from build123d import *

# Parameters (mm, degrees)
F1_DEPTH = 63.5
F0_W     = 25.4
F0_H     = 19.05
F2_DEPTH = 25.4
F3_DEPTH = 7.9375
F5_R     = 5.08


with BuildPart() as f1:
    # F0 (on Front) → F1 (new body, symmetric)
    with BuildSketch(Plane.XZ):
        Polygon((41.275, -9.525), (41.275, 9.525), (22.225, 9.525), (-41.275, 9.525), (-41.275, -9.525), align=None)
    extrude(amount=F1_DEPTH, both=True)

    # F0 (on Front) → F2 (join, symmetric)
    with BuildSketch(Plane.XZ):
        with BuildLine():
            Line((22.225, 9.525), (41.275, 9.525))
            Line((41.275, 9.525), (41.275, 27.0666779783))
            ThreePointArc((41.275, 27.0666779783), (45.3781164095, 37.7174235733), (55.566449667, 42.8625))
            Line((55.566449667, 42.8625), (60.325, 42.8625))
            Line((60.325, 42.8625), (60.325, 61.9125))
            Line((60.325, 61.9125), (54.799614366, 61.9125))
            ThreePointArc((54.799614366, 61.9125), (31.6368382666, 50.9169233306), (22.225, 27.0666779783))
            Line((22.225, 27.0666779783), (22.225, 9.525))
        make_face()
        with Locations((73.025, 52.3875)):
            Rectangle(F0_W, F0_H)
    extrude(amount=F2_DEPTH, both=True)

    # F0 (on Front) → F3 (join, symmetric)
    with BuildSketch(Plane.XZ):
        with BuildLine():
            Line((-41.275, 9.525), (22.225, 9.525))
            Line((22.225, 9.525), (22.225, 27.0666779783))
            ThreePointArc((22.225, 27.0666779783), (31.6368382666, 50.9169233306), (54.799614366, 61.9125))
            add(Edge.make_bspline(
                [(-41.275, 9.525), (-33.6213931441, 35.8969122171), (10.3490389884, 59.2281594872), (54.799614366, 61.9125)],
                knots=[0, 0, 0, 0, 109.4293456154, 109.4293456154, 109.4293456154, 109.4293456154], degree=3))
        make_face()
    extrude(amount=F3_DEPTH, both=True)

    # F0 (on Front) → F4 (revolve)
    with BuildSketch(Plane.XZ):
        Polygon((85.725, 61.9125), (85.725, 42.8625), (85.725, 37.1208467424), (111.125, 37.1208467424), (111.125, 65.6958467424), (85.725, 65.6958467424), align=None)
    revolve(axis=Axis((85.725, 0, 51.4083467424), (0, 0, 1)))

    # F5
    f5_edges = [f1.edges().sort_by_distance(p)[0] for p in [
        (41.275, -63.5, 0),
        (41.275, 63.5, 0),
        (-41.275, -63.5, 0),
        (-41.275, 63.5, 0),
        (41.275, 0, 27.066678),
    ]]
    fillet(f5_edges, radius=F5_R)


solid = f1.part
Could you check a few things on this model? Use its own coordinates, in mm. A direction names the side the tool comes from. Coordinates: 2 decimals unless noted, no trailing zeros. Order: outer loops, then holes, each group sorted by start corner. A loop starts at its lowest first (then second) coordinate and runs counter-clockwise, first axis right, second up. Notation, with made-up numbers: (36.5, 22) - (62.5, 22) arc R24 ccw to (62.5, 32) - close; hole circle Ø11 at (-32.5, -2). An arc over 180 degrees is marked (long way). Answer in a Markdown table with one row per item. Add a question column.
(1) On a 3-axis mill with a long thin cutter (end or side, diameter ignored), from which of +Z, -Z, +X, -X, +Y, -Y can I reach the whole of each face in a straight line? I mean faces 4 (the face through (-5, -7.938, 30)), 5 (the face through (60, 0, 61.912)), 6 (the face through (86, 0, 37.121)), 7 (the face through (22.225, 17, 18)), 8 (the face through (45.269, -0.356, 37.596)). Say none if no direction works.
(2) If we section it at C-C, the plane y = -42.5: Please give me the cut outline in (x, z) (3 decimals), then the cut area to 3 significant figures.
(3) If we section it at A-A, the plane z = -3: Please give me the cut outline in (x, y) (3 decimals).
(4) I need wall thicknesses on L1, parallel to Z at x = 67, y = -3; L2, parallel to Y at x = 11, z = 49; L3, parallel to Y at x = 34, z = 32. Which ranges of each line are inside material? Lowest first, please.
(5) Will these pins go through, and if not, where does the flat tip stop? pin 1 (15.5 mm diameter, centred on x = 22.5, z = 41, fed in from +Y); pin 2 (5 mm diameter, centred on x = -22.5, y = 34.5, fed in from +Z) (3 decimals); pin 3 (19 mm diameter, centred on y = -18, z = 20, fed in from -X) (3 decimals).
(6) If we mould it in two halves opening along X, with no side actions, what happens to faces 1 (the face through (39.8, -62, 0.1)), 2 (the face through (59, 0, 42.862)), 3 (the face through (46, 25.4, 42))? For each: released by +X, released by -X, zero draft, split by the parting line, or undercut.
Results are:
| question | item | result |
|---|---|---|
| 1 | face 4 | +Z, -X, -Y |
| 1 | face 5 | +Z, -X |
| 1 | face 6 | -Z, +X, +Y, -Y |
| 1 | face 7 | +Z, -X, +Y |
| 1 | face 8 | -Z, +Y, -Y |
| 2 | outline | (-41.275, -9.525) - (41.275, -9.525) - (41.275, 9.525) - (-41.275, 9.525) - close |
| 2 | area | 1,570 mm2 |
| 3 | outline | (-41.275, -58.42) arc R5.08 ccw to (-36.195, -63.5) - (36.195, -63.5) arc R5.08 ccw to (41.275, -58.42) - (41.275, 58.42) arc R5.08 ccw to (36.195, 63.5) - (-36.195, 63.5) arc R5.08 ccw to (-41.275, 58.42) - close |
| 4 | L1 | z = 37.12 to 65.7 |
| 4 | L2 | y = -7.94 to 7.94 |
| 4 | L3 | y = -25.4 to 25.4 |
| 5 | pin 1 | stops at y = 25.4 |
| 5 | pin 2 | stops at z = 9.525 |
| 5 | pin 3 | stops at x = 22.225 |
| 6 | face 1 | released by +X |
| 6 | face 2 | undercut |
| 6 | face 3 | zero draft |
